from build123d import *

# Parameters (mm, degrees)
BOSS_EXTRUDE1_START     = -856.54016
SKETCH1_R               = 23.525
SKETCH1_R_2             = 22.525
BOSS_EXTRUDE1_DEPTH     = 40
BOSS_EXTRUDE2_DEPTH     = 40
CUT_EXTRUDE1_DEPTH      = 24.525
CUT_EXTRUDE1_DEPTH_BACK = 24.525


with BuildPart() as part:
    # Sketch1 → Boss-Extrude1 (new body)
    with BuildSketch(Plane.XY.offset(BOSS_EXTRUDE1_START)):
        Circle(SKETCH1_R)
        Circle(SKETCH1_R_2, mode=Mode.SUBTRACT)
    extrude(amount=BOSS_EXTRUDE1_DEPTH)

    # Sketch4 → Boss-Extrude2 (add)
    with BuildSketch(Plane.XY.offset(-816.540159845)):
        Polygon((23.525, -23.525), (23.525, -24.525), (-23.525, -24.525), (-23.525, -23.525), (0, -23.525), align=None)
        with BuildLine():
            Line((23.525, -23.525), (23.525, 0))
            ThreePointArc((23.525, 0), (16.634687027, -16.634687027), (0, -23.525))
            Line((0, -23.525), (23.525, -23.525))
        make_face()
        with BuildLine():
            ThreePointArc((0, -23.525), (-16.634687027, -16.634687027), (-23.525, 0))
            Line((-23.525, 0), (-23.525, -23.525))
            Line((-23.525, -23.525), (0, -23.525))
        make_face()
    extrude(amount=-BOSS_EXTRUDE2_DEPTH)

    # Sketch3 → Cut-Extrude1 (cut, two sides)
    with BuildSketch(Plane(origin=(0, 0, 0), x_dir=(0, 0, -1), z_dir=(1, 0, 0))) as cut_extrude1_sk:
        Polygon((827.542837087, 23.525), (856.540159845, -22.225), (856.540159845, 23.525), align=None)
    extrude(amount=CUT_EXTRUDE1_DEPTH, mode=Mode.SUBTRACT)
    extrude(cut_extrude1_sk.sketch, amount=-CUT_EXTRUDE1_DEPTH_BACK, mode=Mode.SUBTRACT)


solid = part.part
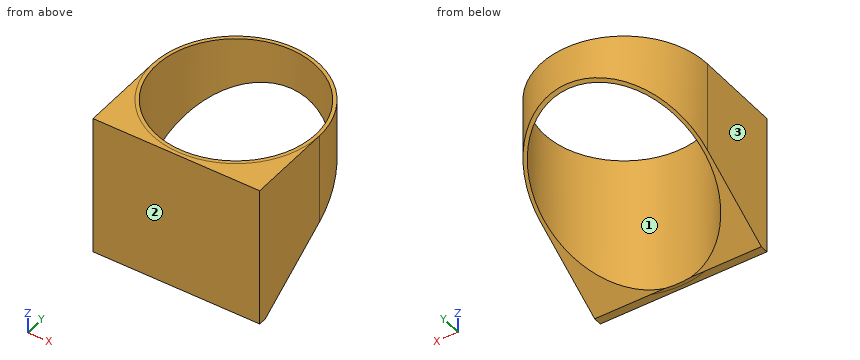
Can you work these out from the model? Positions are in its coordinate system, mm. Face numbers are marked on the shaded views. Coordinates: 2 decimals unless noted, no trailing zeros. Order: outer loops, then holes, each group sorted by start corner. A loop starts at its lowest first (then second) coordinate and runs counter-clockwise, first axis right, second up. Notation, with made-up numbers: (41.25, 1.5) - (47.25, 1.5) arc R10 cw to (47.25, 14.5) - close; hole circle Ø9 at (1.5, -29.5). An arc over 180 degrees is marked (long way). Answer as a JSON object with one key per item and string values. Group by question number.
Q1. Imagine slicing it at A-A (x = -16). Please give me the cut outline in (y, z) (3 decimals), and give its area (3 significant figures).
Q2. Will these pins go through, and if not, where does the flat tip stop? P1, Ø5, axis at y = 5, z = -826, coming from the -X side; P2, Ø5, axis at x = -17, z = -822, coming from the +Y side (3 decimals); P3, Ø1, axis at x = -17.5, z = -829.5, coming from the +Y side.
Q3. I need wall thicknesses on line 1 (X direction, y = 0, z = -837.5) (3 decimals); line 2 (Y direction, x = 0, z = -827) (3 decimals); line 3 (Y direction, x = 0, z = -845) (3 decimals). Which ranges of each line are inside material? Lowest first, please. Write a range as from..to.
Q4. Imagine slicing it at B-B (y = 2.5). Please give me the cut outline in (x, z), and give its area (3 significant figures).
Q5. Imagine slicing it at C-C (z = -819.5). Please give me the cut outline in (x, y) (3 decimals), and give its area (3 significant figures).
Q6. Imagine slicing it at D-D (x = 12). Please give me the cut outline in (y, z) (3 decimals).
Q7. We'd pull the mould along Y, two halves only. Please class the marked faces 1, 2 and 3: +Y half, -Y half, draft (parallel to the pull), parting line (faces both ways), or undercut.
Determined:
{
 "1": {"outline": "(-24.525, -856.54) - (-22.225, -856.54) - (-15.855, -852.503) - (-15.855, -816.54) - (-24.525, -816.54) - close; (15.855, -832.404) - (17.246, -831.523) - (17.246, -816.54) - (15.855, -816.54) - close", "area": "355 mm2"},
 "2": {"P1": "stops at x = -23.39", "P2": "stops at y = 18.525", "P3": "stops at y = 16.26"},
 "3": {"line 1": "x = -23.525..-22.525, 22.525..23.525", "line 2": "y = -24.525..-22.525, 22.525..23.525", "line 3": "y = -24.525..-22.525"},
 "4": {"outline": "(-23.39, -840.87) - (-22.39, -840.87) - (-22.39, -816.54) - (-23.39, -816.54) - close; (22.39, -840.87) - (23.39, -840.87) - (23.39, -816.54) - (22.39, -816.54) - close", "area": "48.9 mm2"},
 "5": {"outline": "(-23.525, -24.525) - (23.525, -24.525) - (23.525, 0) arc R23.525 ccw to (-23.525, 0) - close; hole circle Ø45.05 at (0, 0)", "area": "429 mm2"},
 "6": {"outline": "(-24.525, -856.54) - (-22.225, -856.54) - (-19.062, -854.536) - (-19.062, -816.54) - (-24.525, -816.54) - close; (19.062, -830.371) - (20.234, -829.629) - (20.234, -816.54) - (19.062, -816.54) - close"},
 "7": {"face 1": "undercut", "face 2": "-Y half", "face 3": "draft"}
}
